Work out the finished part from the listing and answer in its coordinate system (mm). Coordinates: 2 decimals unless noted, no trailing zeros. Order: outer loops, then holes, each group sorted by start corner. A loop starts at its lowest first (then second) coordinate and runs counter-clockwise, first axis right, second up. Notation, with made-up numbers: (30, 26.5) -> (67, 26.5) arc R28 cw to (67, 46.5) -> close; hole circle Ø1 at (74, 69.5). An arc over 180 degrees is marked (long way). Use one line per item in the form item = value.
from build123d import *

# Parameters (mm, degrees)
SKETCH_W     = 22
SKETCH_H     = 34.4
PAD_DEPTH    = 1.5
SKETCH001_W  = 26
SKETCH001_H  = 36.4
PAD001_DEPTH = 1
SKETCH002_W  = 8
SKETCH002_H  = 1
POCKET_DEPTH = 1.5


with BuildPart() as part:
    # Sketch → Pad (new body)
    with BuildSketch(Plane.XY):
        Rectangle(SKETCH_W, SKETCH_H)
    extrude(amount=PAD_DEPTH)

    # Sketch001 (on Face6 of Pad) → Pad001 (join)
    with BuildSketch(Plane.XY.offset(1.5)):
        with Locations((0, -1)):
            Rectangle(SKETCH001_W, SKETCH001_H)
    extrude(amount=PAD001_DEPTH)

    # Sketch002 (on Face11 of Pad001) → Pocket (cut)
    with BuildSketch(Plane.XY.offset(2.5)):
        with Locations((0, 16.7)):
            Rectangle(SKETCH002_W, SKETCH002_H)
    extrude(amount=-POCKET_DEPTH, mode=Mode.SUBTRACT)


solid = part.part
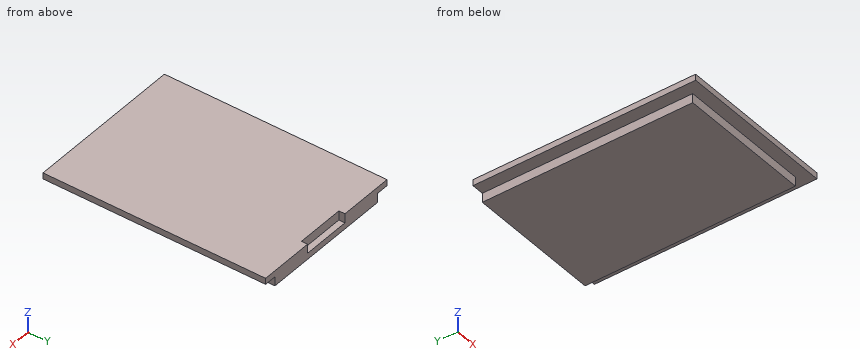
(1) Straight lines are drawn through the part: line 1 along X through (y, z) = (8.5, 0.25); line 2 along Y through (x, z) = (1.75, 1.1); line 3 along Y through (x, z) = (0.75, 1.9). For each, find the intervals that lie inside material, in ascending order.
Data:
line_1 = -11 to 11
line_2 = -17.2 to 16.2
line_3 = -19.2 to 16.2
(2) Section C-C on z = 0.6 is taken. Write down the section's boundary in (x, y).
Data:
outline = (-11, -17.2) -> (11, -17.2) -> (11, 17.2) -> (-11, 17.2) -> close
(3) Section B-B on x = -3.25 is taken. Write down the section's boundary in (y, z), plus the area to 3 significant figures.
Data:
outline = (-19.2, 1.5) -> (-17.2, 1.5) -> (-17.2, 0) -> (17.2, 0) -> (17.2, 1) -> (16.2, 1) -> (16.2, 2.5) -> (-19.2, 2.5) -> close
area = 86.5 mm²
(4) Section A-A on y = -15 is taken. Write down the section's boundary in (x, z), plus the area to 3 significant figures.
Data:
outline = (-13, 1.5) -> (-11, 1.5) -> (-11, 0) -> (11, 0) -> (11, 1.5) -> (13, 1.5) -> (13, 2.5) -> (-13, 2.5) -> close
area = 59.0 mm²
(5) Each of these flat-tipped pins is pushed along its axis until it touches: P1, Ø0.8, axis at y = -3, z = 1, coming from the -X side; P2, Ø0.8, axis at x = -4, z = 1, coming from the -Y side; P3, Ø1.2, axis at x = 0.5, z = 2, coming from the +Y side. Where does it stop, or does it pass through?
Data:
P1 = -11
P2 = -17.2
P3 = 16.2
(6) Section D-D on x = -10 is taken. Write down the section's boundary in (y, z), plus the area to 3 significant figures.
Data:
outline = (-19.2, 1.5) -> (-17.2, 1.5) -> (-17.2, 0) -> (17.2, 0) -> (17.2, 2.5) -> (-19.2, 2.5) -> close
area = 88.0 mm²
